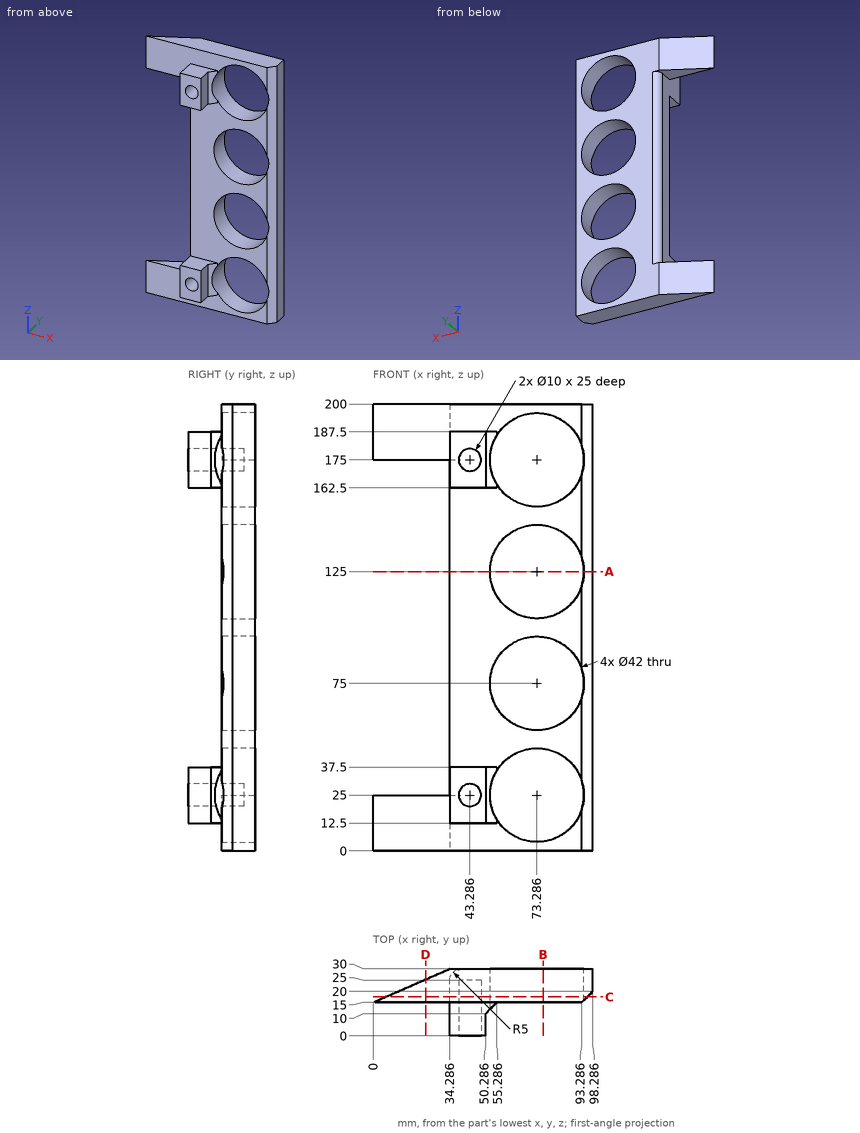
Geometry: see drawing. Coordinates: mm, zero at the bounding-box minimum. Round coordinates to 2 decimals unless told otherwise and drop trailing zeros. Loops run counter-clockwise (first coordinate to the right, second up) from the corner with the lowest first, then second, coordinate; pieces in that order, holes last. Notation, with made-up numbers: M 27.5,-2.75 L 59.5,-2.75 A23 ccw 59.5,8.25 Z; hole C 70,-28.75 d10. An arc over 180 degrees is marked long. Use a Markdown table: item, result. Add a question column.
1. Ray query, line 1 along Z through (x, y) = (57, 28) (1 decimal); line 2 along Z through (x, y) = (74, 27.5); line 3 along Z through (x, y) = (25, 19). Return the intervals inside material, ascending. Write a range as [from, to].
2. Cut plane A-A, the plane z = 125. Output: boundary loops of the cut face in (x, y) (1 decimal).
3. Cut plane B-B, the plane x = 76. Output: boundary loops of the cut face in (y, z), and give its area (3 significant figures).
4. Cut plane D-D, the plane x = 23.5. Output: boundary loops of the cut face in (y, z).
5. Cut plane C-C, the plane y = 17.5. Output: boundary loops of the cut face in (x, z) (1 decimal), and give its area (3 significant figures).
6. Contact query for flat-ended pins moving along their axis: pin 1 (16.5 mm diameter, centred on x = 50, y = 4.5, fed in from +Z); pin 2 (16.5 mm diameter, centred on x = 48, y = 4.5, fed in from -Z); pin 3 (11 mm diameter, centred on y = 7.5, z = 29, fed in from +X). Output: stop coordinate, or through.
Solution:
| question | item | result |
|---|---|---|
| 1 | line 1 | z = [0, 11.7], [38.3, 61.7], [88.3, 111.7], [138.3, 161.7], [188.3, 200] |
| 1 | line 2 | z = [0, 4.01], [45.99, 54.01], [95.99, 104.01], [145.99, 154.01], [195.99, 200] |
| 1 | line 3 | z = [0, 25], [175, 200] |
| 2 | outline | M 34.3,15 L 52.3,15 L 52.3,30 L 39.3,30 A5 ccw 34.3,25 Z; M 94.3,16 L 98.3,20 L 98.3,30 L 94.3,30 Z |
| 3 | outline | M 15,0 L 30,0 L 30,4.18 L 15,4.18 Z; M 15,45.82 L 30,45.82 L 30,54.18 L 15,54.18 Z; M 15,95.82 L 30,95.82 L 30,104.18 L 15,104.18 Z; M 15,145.82 L 30,145.82 L 30,154.18 L 15,154.18 Z; M 15,195.82 L 30,195.82 L 30,200 L 15,200 Z |
| 3 | area | 501 mm2 |
| 4 | outline | M 15,0 L 25.28,0 L 25.28,25 L 15,25 Z; M 15,175 L 25.28,175 L 25.28,200 L 15,200 Z |
| 5 | outline | M 5.7,0 L 95.8,0 L 95.8,200 L 5.7,200 L 5.7,175 L 34.3,175 L 34.3,25 L 5.7,25 Z; hole C 43.3,25 d10; hole C 43.3,175 d10; hole C 73.3,25 d42; hole C 73.3,75 d42; hole C 73.3,125 d42; hole C 73.3,175 d42 |
| 5 | area | 8,030 mm2 |
| 6 | pin 1 | stops at z = 187.5 |
| 6 | pin 2 | stops at z = 12.5 |
| 6 | pin 3 | stops at x = 53.05 |
